Autodesk Inventor part; units mm, degrees
ref_plane "YZ Plane" through (0, 0, 0) normal (1, 0, 0) x (0, 1, 0)
ref_plane "XZ Plane" through (0, 0, 0) normal (0, 1, 0) x (-1, 0, 0)
ref_plane "XY Plane" through (0, 0, 0) normal (0, 0, 1) x (1, 0, 0)
sketch "Sketch1" plane through (0, 0, 0) normal (0, 1, 0) x (-1, 0, 0)
  circle A0 centre (-56.7045, -56.3864) radius 4.8895
  circle A1 centre (-56.7045, -56.3864) radius 4.8895
  line L0 (-52.2143, -60.8765) -> (69.7375, 61.0754)
  line L1 (60.7573, 70.0556) -> (-61.1946, -51.8963)
  arc A2 (-61.1946, -51.8963) -> (-52.2143, -60.8765) centre (-56.7045, -56.3864) ccw
  arc A3 (69.7375, 61.0754) -> (60.7573, 70.0556) centre (65.2474, 65.5655) ccw
  circle A4 centre (4.2715, 4.5895) radius 4.8895
  circle A5 centre (65.2474, 65.5655) radius 4.8895
  line L2 (7.7289, 8.0469) -> (61.79, 62.1081)
  line L3 (68.7048, 69.0229) -> (69.7375, 70.0556)
  line L4 (-53.2471, -52.929) -> (0.8141, 1.1322) construction
  line L5 (7.7289, 8.0469) -> (61.79, 62.1081) construction
  line L6 (0.8141, 1.1322) -> (-53.2471, -52.929)
  line L7 (-60.1619, -59.8438) -> (-61.1946, -60.8765)
  line L8 (-5.0037, -4.6857) -> (-47.4293, -47.1112) construction
  line L9 (-7.5546, -2.1348) -> (-49.9802, -44.5603)
  line L10 (-44.8784, -49.6621) -> (-2.4529, -7.2365)
  arc A6 (-2.4529, -7.2365) -> (-7.5546, -2.1348) centre (-5.0037, -4.6857) ccw
  arc A7 (-49.9802, -44.5603) -> (-44.8784, -49.6621) centre (-47.4293, -47.1112) ccw
  line L11 (4.2715, 4.5895) -> (-0.2187, 9.0797)
  arc A8 (10.9958, 16.4156) -> (16.0976, 11.3139) centre (13.5467, 13.8648) ccw
  line L12 (10.9958, 16.4156) -> (53.4213, 58.8412)
  line L13 (58.5231, 53.7394) -> (16.0976, 11.3139)
  arc A9 (58.5231, 53.7394) -> (53.4213, 58.8412) centre (55.9722, 56.2903) ccw
  line L14 (70.6356, 60.1773) -> (-51.3163, -61.7745)
  arc A10 (-62.0926, -50.9982) -> (-51.3163, -61.7745) centre (-56.7045, -56.3864) ccw
  line L15 (-62.0926, -50.9982) -> (59.8592, 70.9536)
  arc A11 (70.6356, 60.1773) -> (59.8592, 70.9536) centre (65.2474, 65.5655) ccw
  circle A12 centre (65.2474, 65.5655) radius 7.62
  point P0 (0, 0)
  point P1 (29.6663, 4.6577)
  point P2 (-26.2165, -25.8984)
  dimension "d0" = 172.466
  dimension "d1" = 12.7
  dimension "d2" = 9.779
  dimension "d3" = 9.779
  dimension "d4" = 9.779
  dimension "d9" = 1.27
extrude "Extrusion1" add sketch "Sketch1" along normal blind 7.62 contours A0 L6 A7 L10 A6 A4 L2 A8 L13 A9 A12 L0 A2 L7 | A0 L7 A2 L1 L11 A4 L6 A6 L9 A7 | L1 A12 L2 A9 L12 A8 A4 L11 | A12 L2 A5 L3 A3 L0 | L1 A3 L3 A5 L2 A12
sketch "Sketch2" plane through (0, 7.62, 0) normal (0, 1, 0) x (1, 0, 0)
  line L0 (-60.7573, -70.0556) -> (61.1946, 51.8963)
  arc A0 (61.1946, 51.8963) -> (52.2143, 60.8765) centre (56.7045, 56.3864) ccw
  line L1 (52.2143, 60.8765) -> (-69.7375, -61.0754)
  arc A1 (-69.7375, -61.0754) -> (-60.7573, -70.0556) centre (-65.2474, -65.5655) ccw
  arc A2 (-58.5231, -53.7394) -> (-53.4213, -58.8412) centre (-55.9722, -56.2903) ccw
  line L2 (-58.5231, -53.7394) -> (-16.0976, -11.3139)
  arc A3 (-10.9958, -16.4156) -> (-16.0976, -11.3139) centre (-13.5467, -13.8648) ccw
  line L3 (-10.9958, -16.4156) -> (-53.4213, -58.8412)
  circle A4 centre (-65.2474, -65.5655) radius 4.8895
  circle A5 centre (-4.2715, -4.5895) radius 4.8895
  circle A6 centre (56.7045, 56.3864) radius 4.8895
  arc A7 (49.9802, 44.5603) -> (44.8784, 49.6621) centre (47.4293, 47.1112) ccw
  line L4 (49.9802, 44.5603) -> (7.5546, 2.1348)
  arc A8 (2.4529, 7.2365) -> (7.5546, 2.1348) centre (5.0037, 4.6857) ccw
  line L5 (2.4529, 7.2365) -> (44.8784, 49.6621)
  circle A9 centre (-65.2474, -65.5655) radius 6.35
  point P0 (0, 0)
extrude "Extrusion2" add sketch "Sketch2" along normal blind 7.62 contours A1 A9
extrude "Extrusion3" add sketch "Sketch1" along normal blind 7.62 contours A2 L0 A12 L14 A10 L15 L1 | L0 A3 L1 A12 A11
extrude "Extrusion4" add sketch "Sketch1" along normal up to surface (15.24 mm away) contours A12 L2 A5 L3 A3 L0 | L0 A3 L1 A12 A11 | L1 A3 L3 A5 L2 A12 | A5
extrude "Extrusion5" cut sketch "Sketch1" along normal blind 25.4 contours A5
properties part number "Bump Arm"
Work out the finished part from the listing and answer in its coordinate system (mm). A direction names the side the tool comes from. Coordinates: 2 decimals unless noted, no trailing zeros. Write each loop counter-clockwise with the first axis right and the second up, starting at its lowest first coordinate (ties: lowest second). Pieces come first, ordered by that corner, then holes. Notation, with made-up numbers: M -6.75,59.25 L 24.25,59.25 A27 ccw 24.25,98.25 Z; hole C 68,81.5 d4. An arc over 180 degrees is marked long. Use one line per item in the form item = value. Start each with the question number.
1. The part is cut by section A-A (x = 5). Give the vertices of the cut face in (y, z).
2. Straight lines are drawn through the part: probe 1 along Z at (x, y) = (31, 3.75); probe 2 along X at (y, z) = (6.5, -58); probe 3 along X at (y, z) = (3.5, -12.5). For each, find the intervals that lie inside material, in ascending order. Write a range as from..to.
3. The part is cut by section B-B (y = 6). Give the vertices of the cut face in (x, z) (1 decimal), plus the area to 3 significant figures.
4. The part is cut by section D-D (z = 29.5). Give the vertices of the cut face in (x, y), plus the area to 3 significant figures.
5. The mould has two halves that part along X. Classify faces 4 (the face through (61.973, 3.757, -61.892)), 5 (the face through (-9, 0, 0)), 6 (the face through (1.97, 3.757, 9.124)), 7 (the face through (57.764, 3.757, -51.613)): released by +X, released by -X, zero draft, split by the parting line, or undercut.
6. The part is cut by section C-C (z = 63). Give the vertices of the cut face in (x, y), plus the area to 3 significant figures.
7. Each of these flat-tipped pins is pushed along its axis until it touches: P1, Ø4, axis at x = -1.5, y = 4.5, coming from the +Z side; P2, Ø4, axis at y = 5, z = 33, coming from the +X side; P3, Ø1.5, axis at x = -30, z = 42, coming from the +Y side. Where does it stop, or does it pass through?
8. A tool of negligible diameter and unlimited length cuts with its end or side. For faces 1 (the face through (-59.98, 11.38, 60.06)), 2 (the face through (-10.513, 3.757, 0.055)), 3 (the face through (23.963, 3.757, -28.746)), from which of +Z, -Z, +X, -X, +Y, -Y can it reach the whole face along a straight path? Write none if from no direction.
Evaluation:
q1.outline = M 0,-15.46 L 7.62,-15.46 L 7.62,-9.78 L 0,-9.78 Z; M 0,-1.08 L 7.62,-1.08 L 7.62,6.09 L 0,6.09 Z
q2.probe_1 = -41.46..-35.78, -25.58..-19.91
q2.probe_2 = 47.54..52.09, 61.32..64.15
q2.probe_3 = 2.04..7.72, 17.92..23.59
q3.outline = M -70.6,60.2 L 51.3,-61.8 A7.6 ccw 62.1,-51 L -59.9,71 A7.6 ccw Z; hole C -65.2,65.6 d9.8; hole M -58.5,53.7 L -16.1,11.3 A3.6 ccw -11,16.4 L -53.4,58.8 A3.6 ccw Z; hole C -4.3,4.6 d9.8; hole M 2.5,-7.2 L 44.9,-49.7 A3.6 ccw 50,-44.6 L 7.6,-2.1 A3.6 ccw Z; hole C 56.7,-56.4 d9.8
q3.area = 1,640 mm^2
q4.outline = M -39.96,0 L -34.28,0 L -34.28,7.62 L -39.96,7.62 Z; M -24.08,0 L -18.41,0 L -18.41,7.62 L -24.08,7.62 Z
q4.area = 86.5 mm^2
q5.face_4 = split by the parting line
q5.face_5 = zero draft
q5.face_6 = released by +X
q5.face_7 = undercut
q6.outline = M -72.42,0 L -69.41,0 L -69.41,15.24 L -72.42,15.24 Z; M -61.09,0 L -51.91,0 L -51.91,7.62 L -58.07,7.62 L -58.07,15.24 L -61.09,15.24 Z
q6.area = 139 mm^2
q7.P1 = 14.59
q7.P2 = -19.91
q7.P3 = 7.62
q8.face_1 = +Y
q8.face_2 = -Z, -X, +Y, -Y
q8.face_3 = +Y, -Y
